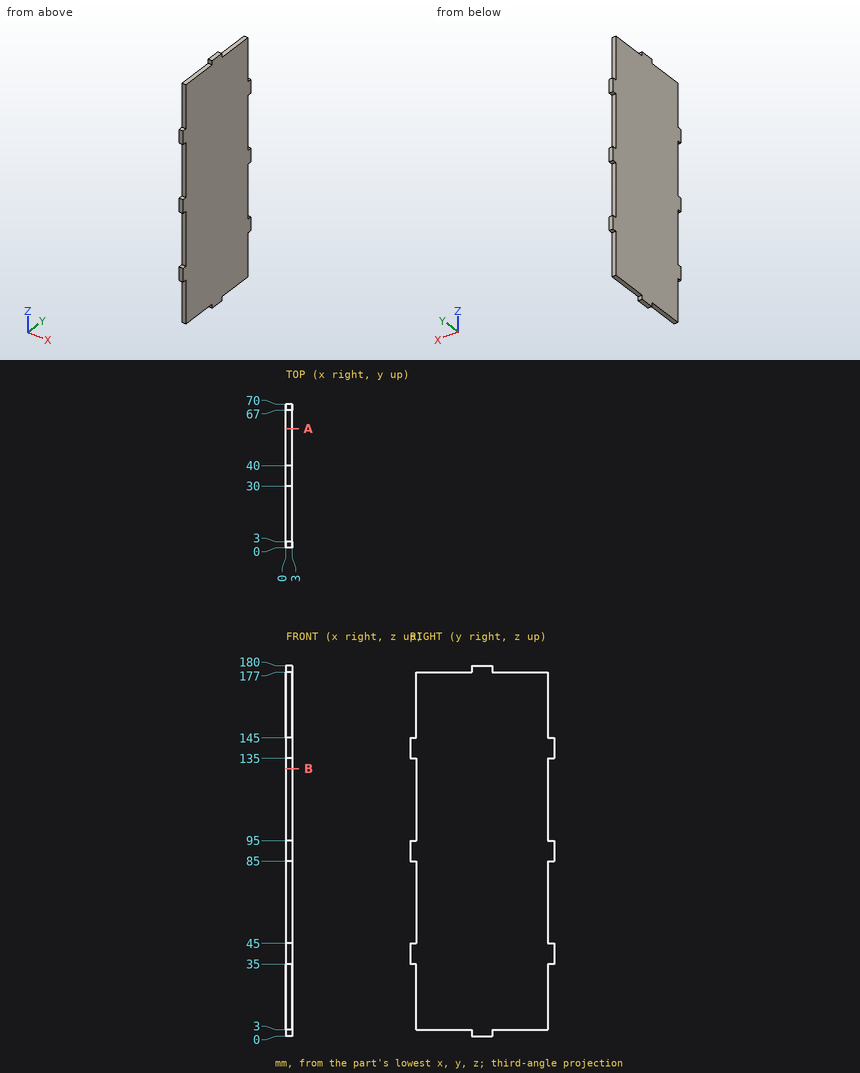
Here's the drawing with two shaded views (mm, measured from the low corner). I have some questions. Coordinates: 2 decimals unless noted, no trailing zeros. Write each loop counter-clockwise with the first axis right and the second up, starting at its lowest first coordinate (ties: lowest second). Pieces come first, ordered by that corner, then holes. Notation, with made-up numbers: (77, -11) - (115, -11) arc R36 cw to (115, 28) - close; hole circle Ø2 at (50, 67.25). An arc over 180 degrees is marked (long way). Return JSON: item names as keys, results as strings.
Q1. If we section it at B-B (z = 130): Please give me the cut outline in (x, y), then the cut area to 3 significant figures.
Computed values:
{"outline": "(0, 3) - (3, 3) - (3, 67) - (0, 67) - close", "area": "192 mm2"}
Q2. If we section it at A-A (y = 58): Please give me the cut outline in (x, z).
Computed values:
{"outline": "(0, 3) - (3, 3) - (3, 177) - (0, 177) - close"}
Q3. Please list where these lines run through material, in increasing order: L1, parallel to Y at x = 1.75, z = 76; L2, parallel to Z at x = 0.6, y = 63. Write a range as from..to.
Computed values:
{"L1": "y = 3..67", "L2": "z = 3..177"}
Q4. I'm going to push flat-ended pins straight in: pin 1 Ø0.9 at (x, y) = (2, 60) entering from +Z; pin 2 Ø1.5 at (x, y) = (1, 68) entering from +Z; pin 3 Ø1.5 at (x, z) = (1, 131.5) entering from -Y; pin 4 Ø8 at (y, z) = (24, 103) entering from -X. Where does each tip first touch, or does it pass through?
Computed values:
{"pin 1": "stops at z = 177", "pin 2": "stops at z = 145", "pin 3": "stops at y = 3", "pin 4": "stops at x = 0"}
